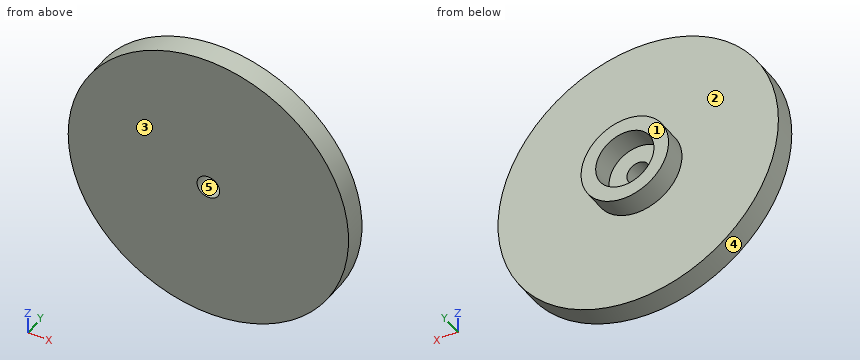
Autodesk Inventor part; units mm, degrees
ref_plane "YZ Plane" through (0, 0, 0) normal (1, 0, 0) x (0, 1, 0)
ref_plane "XZ Plane" through (0, 0, 0) normal (0, 1, 0) x (-1, 0, 0)
ref_plane "XY Plane" through (0, 0, 0) normal (0, 0, 1) x (1, 0, 0)
sketch "Boceto1" plane through (0, 0, 0) normal (0, 1, 0) x (-1, 0, 0)
  circle A0 centre (0, 0) radius 12.51
  dimension "d0" = 25.02
extrude "Extrusión1" add sketch "Boceto1" along normal blind 2
sketch "Boceto2" plane through (0, 2, 0) normal (0, 1, 0) x (1, 0, 0)
  circle A0 centre (0, 0) radius 12.51
  circle A1 centre (0, 0) radius 3.905
  dimension "d3" = 7.81
extrude "Extrusión2" add sketch "Boceto2" along normal blind 2 contours A1
hole "Hole1" at (0, 4, 0) direction (0, -1, 0) diameter 5.2 depth 2
hole "Hole2" at (0, 2, 0) direction (0, -1, 0) diameter 2.02 end through all
properties part number "TapaFrontal"
Input: part model. Units: mm. Frame: model coordinates. Face numbers are marked on the shaded views. A direction names the side the tool comes from. Coordinates: 2 decimals unless noted, no trailing zeros. Loops run counter-clockwise (first coordinate to the right, second up) from the corner with the lowest first, then second, coordinate; pieces in that order, holes last.
Q1. Draft query along Z for the marked faces 3, 4 and 5. Return one class per face: +Z half, -Z half, draft (parallel to the pull), parting line (faces both ways), or undercut.
Q2. Cut plane C-C (y = 3). Output: boundary loops of the cut face in (x, z) (3 decimals).
Q3. Cut plane B-B (x = 0). Output: boundary loops of the cut face in (y, z) (3 decimals), then the cut area to 3 significant figures.
Q4. Set-up query: the marked faces 1 and 2. Return all of +Z, -Z, +X, -X, +Y, -Y with unobstructed straight access to the full face (end or side cutting, diameter ignored); none if empty.
Q5. Contact query for flat-ended pins moving along their axis: pin 1 (2 mm diameter, centred on x = -7, z = -8, fed in from +Y); pin 2 (1.6 mm diameter, centred on x = 0, z = 0, fed in from -Y). Output: stop coordinate, or through.
Q6. Material intervals for line 1 (Z direction, x = 0, y = 3.55) (3 decimals); line 2 (Z direction, x = 0, y = 0.6), sorted ascending.
Q7. Cut plane D-D (y = 1.35). Output: boundary loops of the cut face in (x, z).
Q8. Cut plane A-A (z = 0). Output: boundary loops of the cut face in (x, y) (3 decimals).
Working result:
1. face 3: draft
1. face 4: parting line
1. face 5: undercut
2. outline: circle Ø7.81 at (0, 0); hole circle Ø5.2 at (0, 0)
3. outline: (0, -12.51) - (2, -12.51) - (2, -3.905) - (4, -3.905) - (4, -2.6) - (2, -2.6) - (2, -1.01) - (0, -1.01) - close; (0, 1.01) - (2, 1.01) - (2, 2.6) - (4, 2.6) - (4, 3.905) - (2, 3.905) - (2, 12.51) - (0, 12.51) - close
3. area: 51.2 mm2
4. face 1: +Z, -Z, +X, -X, +Y
4. face 2: +Y
5. pin 1: stops at y = 2
5. pin 2: passes through
6. line 1: z = -3.905 to -2.6, 2.6 to 3.905
6. line 2: z = -12.51 to -1.01, 1.01 to 12.51
7. outline: circle Ø25.02 at (0, 0); hole circle Ø2.02 at (0, 0)
8. outline: (-12.51, 0) - (-1.01, 0) - (-1.01, 2) - (-2.6, 2) - (-2.6, 4) - (-3.905, 4) - (-3.905, 2) - (-12.51, 2) - close; (1.01, 0) - (12.51, 0) - (12.51, 2) - (3.905, 2) - (3.905, 4) - (2.6, 4) - (2.6, 2) - (1.01, 2) - close
